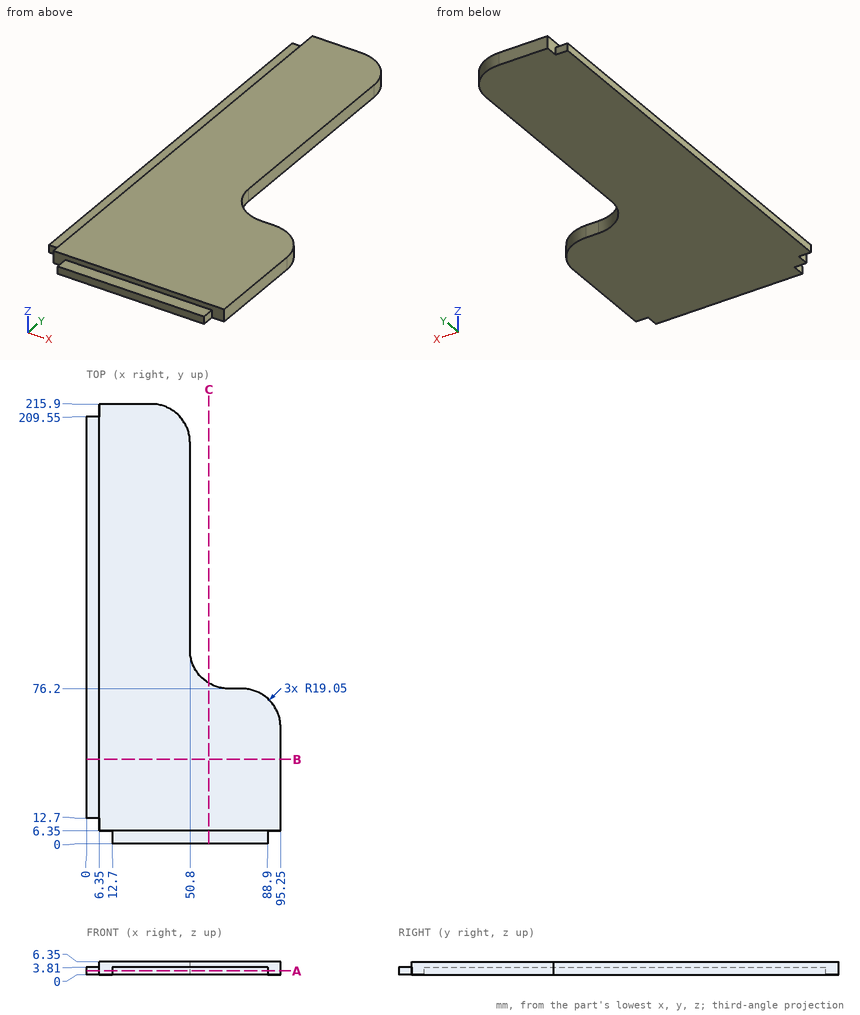
Geometry: see drawing. Coordinates: mm, zero at the bounding-box minimum. Coordinates: 2 decimals unless noted, no trailing zeros. Order: outer loops, then holes, each group sorted by start corner. A loop starts at its lowest first (then second) coordinate and runs counter-clockwise, first axis right, second up. Notation, with made-up numbers: M -15.5,42 L 8.5,42 A36 cw 8.5,77 Z; hole C 22.25,29 d11. An arc over 180 degrees is marked long. Answer in a Markdown table with one row per item. Add a question column.
Q1. Line query: L1, parallel to X at y = 117.5, z = 2.5; L2, parallel to Y at x = 70.5, z = 0.75; L3, parallel to X at y = 55.5, z = 5.5. Output: solid intervals per line, ascending.
Q2. Section query A-A on z = 2. Return the cut outline in (x, y), and give its area (3 significant figures).
Q3. Section query C-C on x = 60. Return the cut outline in (y, z).
Q4. Section query B-B on y = 41.5. Return the cut outline in (x, z).
Q5. Contact query for flat-ended pins moving along their axis: P1, Ø3, axis at y = 2, z = 3, coming from the +X side; P2, Ø3, axis at x = 74, z = 3.5, coming from the +Y side; P3, Ø2, axis at y = 138.5, z = 2, coming from the +X side. Output: stop coordinate, or through.
Completed:
| question | item | result |
|---|---|---|
| 1 | L1 | x = 0 to 50.8 |
| 1 | L2 | y = 0 to 76.2 |
| 1 | L3 | x = 6.35 to 95.25 |
| 2 | outline | M 0,12.7 L 6.35,12.7 L 6.35,6.35 L 12.7,6.35 L 12.7,0 L 88.9,0 L 88.9,6.35 L 95.25,6.35 L 95.25,57.15 A19.05 ccw 76.2,76.2 L 69.85,76.2 A19.05 cw 50.8,95.25 L 50.8,196.85 A19.05 ccw 31.75,215.9 L 6.35,215.9 L 6.35,209.55 L 0,209.55 Z |
| 2 | area | 14,100 mm2 |
| 3 | outline | M 0,0 L 78.94,0 L 78.94,6.35 L 6.35,6.35 L 6.35,3.81 L 0,3.81 Z |
| 4 | outline | M 0,0 L 95.25,0 L 95.25,6.35 L 6.35,6.35 L 6.35,3.81 L 0,3.81 Z |
| 5 | P1 | stops at x = 88.9 |
| 5 | P2 | stops at y = 76.2 |
| 5 | P3 | stops at x = 50.8 |
